from build123d import *

# Parameters (mm, degrees)
IZIM2_R                                        = 44
Y_KSEKLIK_EKSTR_ZYON1_DEPTH                    = 48
IZIM3_R                                        = 11
KES_EKSTR_ZYON1_DEPTH                          = 35
SERVO_MOTOR_BO_LU_U_REACH                      = 15
IZIM5_R                                        = 5.5
IZIM5_W                                        = 20
IZIM5_H                                        = 6.5
IZIM5_W_2                                      = 6
IZIM5_H_2                                      = 7.2
IZIM6_W                                        = 120
IZIM6_H                                        = 25
KES_EKSTR_ZYON3_DEPTH                          = 49
IZIM7_W                                        = 34
IZIM7_H                                        = 10
KES_EKSTR_ZYON4_DEPTH                          = 37.5
IZIM8_R                                        = 5.5
IZIM8_W                                        = 20
IZIM8_H                                        = 6.5
KES_EKSTR_ZYON5_DEPTH                          = 14
M2_D_Z_BA_L_MAKINE_VIDAS_IN_HAV_A1_D           = 2
M2_D_Z_BA_L_MAKINE_VIDAS_IN_HAV_A1_DEPTH       = 3
M2_D_Z_BA_L_MAKINE_VIDAS_IN_HAV_A1_CSINK_D     = 2.6
M2_D_Z_BA_L_MAKINE_VIDAS_IN_HAV_A1_CSINK_ANGLE = 90
IZIM11_R                                       = 47.5
KES_EKSTR_ZYON6_DEPTH                          = 8.16
IZIM14_R                                       = 47.5
KES_EKSTR_ZYON7_DEPTH                          = 10
IZIM13_R                                       = 7.5
TABAN_AYAKLAR_DEPTH                            = 10
DAIRESEL_KAPLAMA1_COUNT                        = 3
F_3_8_Z_VANA_IN_BORU_Z_VANA_MATKAB_1_D         = 2.286
F_3_8_Z_VANA_IN_BORU_Z_VANA_MATKAB_1_DEPTH     = 10
IZIM18_R                                       = 1.2
KES_EKSTR_ZYON8_DEPTH                          = 10


with BuildPart() as part:
    # Çizim2 → Yükseklik-Ekstrüzyon1 (new body)
    with BuildSketch(Plane(origin=(0, 0, 0), x_dir=(1, 0, 0), z_dir=(0, 1, 0))):
        Circle(IZIM2_R)
    extrude(amount=Y_KSEKLIK_EKSTR_ZYON1_DEPTH)

    # Çizim3 → Kes-Ekstrüzyon1 (cut)
    with BuildSketch(Plane(origin=(0, 48, 0), x_dir=(1, 0, 0), z_dir=(0, 1, 0))):
        Circle(IZIM3_R)
        Polygon((-14, -2), (14, -2), (17, -2), (17, -39.5), (-17, -39.5), (-17, -2), align=None)
        with BuildLine():
            Line((-8, 11.5), (8, 11.5))
            ThreePointArc((8, 11.5), (12.242640687, 9.742640687), (14, 5.5))
            Line((14, 5.5), (14, -2))
            Line((14, -2), (-14, -2))
            Line((-14, -2), (-14, 5.5))
            ThreePointArc((-14, 5.5), (-12.242640687, 9.742640687), (-8, 11.5))
        make_face()
        with BuildLine():
            ThreePointArc((11, 0), (-1.004193186, 10.954067557), (-10.816653826, -2))
            Line((-10.816653826, -2), (10.816653826, -2))
            ThreePointArc((10.816653826, -2), (10.954067557, -1.004193186), (11, 0))
        make_face()
        with BuildLine():
            Line((10.816653826, -2), (-10.816653826, -2))
            ThreePointArc((-10.816653826, -2), (0, -11), (10.816653826, -2))
        make_face()
    extrude(amount=-KES_EKSTR_ZYON1_DEPTH, mode=Mode.SUBTRACT)

    # Çizim5 → Servo Motor Boşluğu (cut, up to next)
    with BuildSketch(Plane(origin=(0, 13, 0), x_dir=(1, 0, 0), z_dir=(0, 1, 0)), mode=Mode.PRIVATE) as servo_motor_bo_lu_u_sk1:
        Circle(IZIM5_R)
    servo_motor_bo_lu_u_tool1 = extrude(servo_motor_bo_lu_u_sk1.sketch, amount=-SERVO_MOTOR_BO_LU_U_REACH, mode=Mode.PRIVATE) & part.part
    add(servo_motor_bo_lu_u_tool1.solids().sort_by_distance((0, 13, 0))[0], mode=Mode.SUBTRACT)
    # Çizim5 → Servo Motor Boşluğu (cut, up to next)
    with BuildSketch(Plane(origin=(0, 13, 0), x_dir=(1, 0, 0), z_dir=(0, 1, 0)), mode=Mode.PRIVATE) as servo_motor_bo_lu_u_sk2:
        with Locations((0, -16.35)):
            Rectangle(IZIM5_W, IZIM5_H)
    servo_motor_bo_lu_u_tool2 = extrude(servo_motor_bo_lu_u_sk2.sketch, amount=-SERVO_MOTOR_BO_LU_U_REACH, mode=Mode.PRIVATE) & part.part
    add(servo_motor_bo_lu_u_tool2.solids().sort_by_distance((0, 13, 16.35))[0], mode=Mode.SUBTRACT)
    # Çizim5 → Servo Motor Boşluğu (cut, up to next)
    with BuildSketch(Plane(origin=(0, 13, 0), x_dir=(1, 0, 0), z_dir=(0, 1, 0)), mode=Mode.PRIVATE) as servo_motor_bo_lu_u_sk3:
        with Locations((-8, -29.9)):
            Rectangle(IZIM5_W_2, IZIM5_H_2)
    servo_motor_bo_lu_u_tool3 = extrude(servo_motor_bo_lu_u_sk3.sketch, amount=-SERVO_MOTOR_BO_LU_U_REACH, mode=Mode.PRIVATE) & part.part
    add(servo_motor_bo_lu_u_tool3.solids().sort_by_distance((-8, 13, 29.9))[0], mode=Mode.SUBTRACT)
    # Çizim5 → Servo Motor Boşluğu (cut, up to next)
    with BuildSketch(Plane(origin=(0, 13, 0), x_dir=(1, 0, 0), z_dir=(0, 1, 0)), mode=Mode.PRIVATE) as servo_motor_bo_lu_u_sk4:
        with Locations((8, -29.9)):
            Rectangle(IZIM5_W_2, IZIM5_H_2)
    servo_motor_bo_lu_u_tool4 = extrude(servo_motor_bo_lu_u_sk4.sketch, amount=-SERVO_MOTOR_BO_LU_U_REACH, mode=Mode.PRIVATE) & part.part
    add(servo_motor_bo_lu_u_tool4.solids().sort_by_distance((8, 13, 29.9))[0], mode=Mode.SUBTRACT)

    # Çizim6 → Kes-Ekstrüzyon3 (cut, through all)
    with BuildSketch(Plane(origin=(0, 48, 0), x_dir=(1, 0, 0), z_dir=(0, 1, 0))):
        with Locations((0, -52)):
            Rectangle(IZIM6_W, IZIM6_H)
    extrude(amount=-KES_EKSTR_ZYON3_DEPTH, mode=Mode.SUBTRACT)

    # Çizim7 → Kes-Ekstrüzyon4 (cut)
    with BuildSketch(Plane.XY.offset(39.5)):
        with Locations((0, 5)):
            Rectangle(IZIM7_W, IZIM7_H)
    extrude(amount=-KES_EKSTR_ZYON4_DEPTH, mode=Mode.SUBTRACT)

    # Çizim8 → Kes-Ekstrüzyon5 (cut, through all)
    with BuildSketch(Plane(origin=(0, 13, 0), x_dir=(1, 0, 0), z_dir=(0, 1, 0))):
        Circle(IZIM8_R)
        with BuildLine():
            Line((14, -2), (11, -2))
            Line((11, -2), (-11, -2))
            Line((-11, -2), (-14, -2))
            Line((-14, -2), (-14, 5.5))
            ThreePointArc((-14, 5.5), (-12.242640687, 9.742640687), (-8, 11.5))
            Line((-8, 11.5), (8, 11.5))
            ThreePointArc((8, 11.5), (12.242640687, 9.742640687), (14, 5.5))
            Line((14, 5.5), (14, -2))
        make_face()
        with BuildLine():
            Line((-5.123475383, -2), (-11, -2))
            Line((-11, -2), (-11, -26.3))
            Line((-11, -26.3), (-5, -26.3))
            Line((-5, -26.3), (-5, -33.5))
            Line((-5, -33.5), (-11, -33.5))
            Line((-11, -33.5), (-11, -39.5))
            Line((-11, -39.5), (11, -39.5))
            Line((11, -39.5), (11, -33.5))
            Line((11, -33.5), (5, -33.5))
            Line((5, -33.5), (5, -26.3))
            Line((5, -26.3), (11, -26.3))
            Line((11, -26.3), (11, -2))
            Line((11, -2), (5.123475383, -2))
            ThreePointArc((5.123475383, -2), (0, -5.5), (-5.123475383, -2))
        make_face()
        with Locations((0, -16.35)):
            Rectangle(IZIM8_W, IZIM8_H, mode=Mode.SUBTRACT)
        with BuildLine():
            ThreePointArc((5.5, 0), (-1.017567048, 5.405049242), (-5.123475383, -2))
            Line((-5.123475383, -2), (5.123475383, -2))
            ThreePointArc((5.123475383, -2), (5.405049242, -1.017567048), (5.5, 0))
        make_face()
        with BuildLine():
            Line((5.123475383, -2), (-5.123475383, -2))
            ThreePointArc((-5.123475383, -2), (0, -5.5), (5.123475383, -2))
        make_face()
    extrude(amount=-KES_EKSTR_ZYON5_DEPTH, mode=Mode.SUBTRACT)

    # M2 Düz Başlı Makine Vidası İçin Havşa1
    with Locations(Plane(origin=(-13.5, 10, 31.5), x_dir=(-1, 0, 0), z_dir=(0, -1, 0))):
        with Locations((0, 0), (0, 8), (0, 16), (0, 24), (-27, 0), (-27, 8), (-27, 16), (-27, 24)):
            CounterSinkHole(M2_D_Z_BA_L_MAKINE_VIDAS_IN_HAV_A1_D / 2, M2_D_Z_BA_L_MAKINE_VIDAS_IN_HAV_A1_CSINK_D / 2, depth=M2_D_Z_BA_L_MAKINE_VIDAS_IN_HAV_A1_DEPTH, counter_sink_angle=M2_D_Z_BA_L_MAKINE_VIDAS_IN_HAV_A1_CSINK_ANGLE)

    # Çizim11 → Kes-Ekstrüzyon6 (cut)
    with BuildSketch(Plane(origin=(0, 48, 0), x_dir=(1, 0, 0), z_dir=(0, 1, 0))):
        Circle(IZIM11_R)
    extrude(amount=-KES_EKSTR_ZYON6_DEPTH, mode=Mode.SUBTRACT)

    # Çizim14 → Kes-Ekstrüzyon7 (cut)
    with BuildSketch(Plane.XZ):
        Circle(IZIM14_R)
    extrude(amount=-KES_EKSTR_ZYON7_DEPTH, mode=Mode.SUBTRACT)

    # Çizim13 → Taban Ayakları (add)
    with BuildSketch(Plane.XZ):
        with Locations((0, -30)):
            Circle(IZIM13_R)
    taban_ayaklar = extrude(amount=-TABAN_AYAKLAR_DEPTH)

    # Dairesel Kaplama1: Taban Ayakları ×3 about axis
    dairesel_kaplama1_axis = Axis((0, 0, 0), (0, 1, 0))
    for i in range(1, DAIRESEL_KAPLAMA1_COUNT):
        add(taban_ayaklar.rotate(dairesel_kaplama1_axis, i * 360 / DAIRESEL_KAPLAMA1_COUNT))

    # 3/8 Zıvana İçin Boru Zıvana Matkabı1
    with Locations(Plane(origin=(-6.731, 39.84, -30), x_dir=(0, 0, 1), z_dir=(0, 1, 0))):
        with Locations((0, 0), (0, 13.462), (38.269, -19.249762114), (51.731, -19.249762114), (38.269, 32.711762114), (51.731, 32.711762114)):
            Hole(F_3_8_Z_VANA_IN_BORU_Z_VANA_MATKAB_1_D / 2, depth=F_3_8_Z_VANA_IN_BORU_Z_VANA_MATKAB_1_DEPTH)

    # Çizim18 → Kes-Ekstrüzyon8 (cut)
    with BuildSketch(Plane(origin=(0, 39.84, 0), x_dir=(1, 0, 0), z_dir=(0, 1, 0))):
        with Locations((-19.5, -5.5)):
            Circle(IZIM18_R)
        with Locations((-19.5, -33.5)):
            Circle(IZIM18_R)
        with Locations((19.5, -5.5)):
            Circle(IZIM18_R)
        with Locations((19.5, -33.5)):
            Circle(IZIM18_R)
    extrude(amount=-KES_EKSTR_ZYON8_DEPTH, mode=Mode.SUBTRACT)


solid = part.part
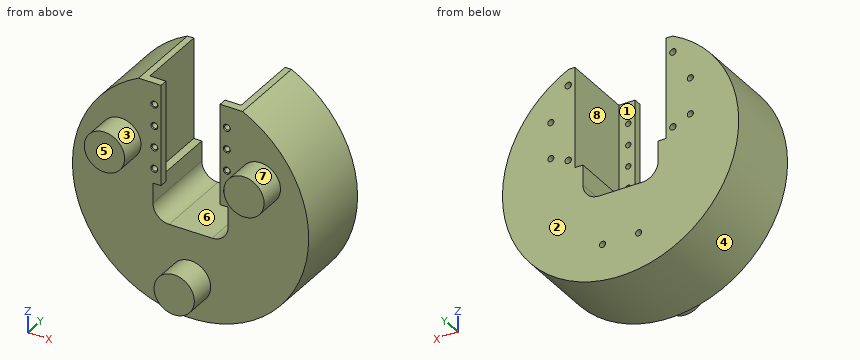
Geometry: final body of the model. Coordinates: model frame, mm. Face numbers are marked on the shaded views. A direction names the side the tool comes from. Give positions to 0.01 mm unless a question says otherwise; leave off trailing zeros. Loops run counter-clockwise (first coordinate to the right, second up) from the corner with the lowest first, then second, coordinate; pieces in that order, holes last. Notation, with made-up numbers: M 19.5,83.5 L 68.5,83.5 A30 cw 68.5,111.5 Z; hole C -29.75,81.25 d8. An arc over 180 degrees is marked long. Put each result on its own line as item: value. Start each with the question number.
1) Cut plane C-C (x = 32). Output: boundary loops of the cut face in (y, z), then the cut area to 3 significant figures.
2) Ray query, line 1 along Z through (x, y) = (-13.5, 12.15); line 2 along Z through (x, y) = (-13, 12); line 3 along X through (y, z) = (10.9, 7.5). Return the intervals inside material, ascending.
3) Contact query for flat-ended pins moving along their axis: pin 1 (2.5 mm diameter, centred on x = -12.5, y = 11, fed in from -Z); pin 2 (12 mm diameter, centred on y = 5, z = 2.5, fed in from -X); pin 3 (5 mm diameter, centred on x = -14.5, z = 1.5, fed in from -Y). Output: stop coordinate, or through.
4) Cut plane B-B (y = 28.5). Output: boundary loops of the cut face in (x, z), then the cut area to 3 significant figures.
5) Access query for the marked faces 5, 6, 7 and 8. Directions: +Z, -Z, +X, -X, +Y, -Y. A direction counts if a zero-diameter tool reaches every point of the face in a straight line with its end or side. Return the directions, or none.
6) Pull-direction query (X, two-part tool) for the marked faces 1, 2, 3 and 4; classes: pulls with the +X half, pulls with the -X half, needs draft (parallel to the pull), parting line crosses it, or undercut.
7) Cut plane A-A (z = 27.5). Output: boundary loops of the cut face in (x, y), then the cut area to 3 significant figures.
8) Cut plane D-D (y = 34.5). Give the number of separate pieces and of enclosed holes in the cut face, then the cut area to 3 significant figures.
Verdict:
1. outline: M 0,10.53 L 10,10.53 L 10,-30.2 L 39.84,-30.2 L 39.84,30.2 L 10,30.2 L 10,19.47 L 0,19.47 Z
1. area: 1,890 mm2
2. line 1: -41.88 to -7.9, 2 to 6.5, 8.5 to 14.5, 16.5 to 22.5, 24.5 to 30.5, 32.5 to 39.5
2. line 2: -42.04 to -8.82, 2 to 6.63, 8.37 to 14.63, 16.37 to 22.63, 24.37 to 30.63, 32.37 to 39.5
2. line 3: -43.36 to -14.5, -12.5 to -11, 11 to 12.5, 14.5 to 43.36
3. pin 1: z = -42.54
3. pin 2: x = -44
3. pin 3: y = 10
4. outline: M -19.38,39.5 A44 ccw long 19.38,39.5 L 17,39.5 L 17,2 L 14,2 L 14,-5.5 A6 cw 8,-11.5 L -8,-11.5 A6 cw -14,-5.5 L -14,2 L -17,2 L -17,39.5 Z
4. area: 4,330 mm2
5. face 5: +Z, -Z, +X, -X, -Y
5. face 6: +Z, +Y, -Y
5. face 7: -Y
5. face 8: +Z, +Y
6. face 1: undercut
6. face 2: needs draft
6. face 3: undercut
6. face 4: parting line crosses it
7. outline: M -34.35,10 L -11,10 L -11,13 L -17,13 L -17,39.84 L -34.35,39.84 Z; M 11,10 L 34.35,10 L 34.35,39.84 L 17,39.84 L 17,13 L 11,13 Z
7. area: 1,070 mm2
8. separate pieces: 1
8. enclosed holes: 10
8. area: 4,280 mm2
